Check sheet for the modelled part. Datum: model origin and axes. Units: mm. A direction names the side the tool comes from. Give positions to 0.01 mm unless a question says otherwise; leave off trailing zeros. Order: outer loops, then holes, each group sorted by start corner. A loop starts at its lowest first (then second) coordinate and runs counter-clockwise, first axis right, second up.
from build123d import *

# Parameters (mm, degrees)
F0_W      = 1600.2
F0_H      = 685.8
F1_DEPTH  = 19.05
F3_DEPTH  = 152.4
F5_DEPTH  = 152.4
F6_W      = 762
F6_H      = 19.05
F7_DEPTH  = 152.4
F8_W      = 381
F8_H      = 19.05
F9_DEPTH  = 152.4
F10_W     = 381
F10_H     = 19.05
F11_DEPTH = 152.4


with BuildPart() as f1:
    # F0 (on Front) → F1 (new body)
    with BuildSketch(Plane.XZ):
        with Locations((800.1, 342.9)):
            Rectangle(F0_W, F0_H)
    extrude(amount=F1_DEPTH)

    # F2 (on face) → F3 (join)
    with BuildSketch(Plane.XZ.offset(19.05)):
        Polygon((0, 685.8), (0, 0), (19.05, 0), (19.05, 666.75), (1581.15, 666.75), (1581.15, 0), (1600.2, 0), (1600.2, 685.8), align=None)
    extrude(amount=F3_DEPTH)

    # F4 (on face) → F5 (join)
    with BuildSketch(Plane.XZ.offset(19.05)):
        Polygon((419.1, 0), (419.1, 666.75), (400.05, 666.75), (400.05, 19.05), (19.05, 19.05), (19.05, 0), align=None)
        Polygon((1200.15, 666.75), (1181.1, 666.75), (1181.1, 0), (1581.15, 0), (1581.15, 19.05), (1200.15, 19.05), align=None)
    extrude(amount=F5_DEPTH)

    # F6 (on face) → F7 (join)
    with BuildSketch(Plane.XZ.offset(19.05)):
        with Locations((800.1, 466.725)):
            Rectangle(F6_W, F6_H)
    extrude(amount=F7_DEPTH)

    # F8 (on face) → F9 (join)
    with BuildSketch(Plane.XZ.offset(19.05)):
        with Locations((209.55, 454.025)):
            Rectangle(F8_W, F8_H)
        with Locations((209.55, 231.775)):
            Rectangle(F8_W, F8_H)
    extrude(amount=F9_DEPTH)

    # F10 (on face) → F11 (join)
    with BuildSketch(Plane.XZ.offset(19.05)):
        with Locations((1390.65, 454.025)):
            Rectangle(F10_W, F10_H)
        with Locations((1390.65, 231.775)):
            Rectangle(F10_W, F10_H)
    extrude(amount=F11_DEPTH)


solid = f1.part
1) Draft check along X on faces 1 (the face through (1388, -94, 666.75)), 2 (the face through (0, -85, 348)), 3 (the face through (789, 0, 348)). Enter one of: +X half, -X half, draft (parallel to the pull), parting line (faces both ways), or undercut.
Recorded:
face 1: undercut
face 2: -X half
face 3: draft
2) Section check B-B, the plane x = 367.5. Record the cut outline in (y, z), then the cut area to 3 significant figures.
Recorded:
outline: (-171.45, 0) - (0, 0) - (0, 685.8) - (-171.45, 685.8) - (-171.45, 666.75) - (-19.05, 666.75) - (-19.05, 463.55) - (-171.45, 463.55) - (-171.45, 444.5) - (-19.05, 444.5) - (-19.05, 241.3) - (-171.45, 241.3) - (-171.45, 222.25) - (-19.05, 222.25) - (-19.05, 19.05) - (-171.45, 19.05) - close
area: 24,700 mm2
3) Section check C-C, the plane y = -48.5. State how many separate pieces and enclosed holes the cut face has, then the cut area to 3 significant figures.
Recorded:
separate pieces: 1
enclosed holes: 7
area: 139,000 mm2
4) Set-up check for faces 4 (the face through (1581.15, -94, 122)), 5 (the face through (789, -8, 0)), 6 (the face through (1181.1, -94, 232)): record each of +Z, -Z, +X, -X, +Y, -Y from which the full face is reachable in a straight line by a thin tool's end or side.
Recorded:
face 4: -Y
face 5: -Z, +X, -X, +Y, -Y
face 6: -Z, -Y
5) Section check A-A, the plane z = 518. Record the cut outline in (x, y), then the cut area to 3 significant figures.
Recorded:
outline: (0, -171.45) - (19.05, -171.45) - (19.05, -19.05) - (400.05, -19.05) - (400.05, -171.45) - (419.1, -171.45) - (419.1, -19.05) - (1181.1, -19.05) - (1181.1, -171.45) - (1200.15, -171.45) - (1200.15, -19.05) - (1581.15, -19.05) - (1581.15, -171.45) - (1600.2, -171.45) - (1600.2, 0) - (0, 0) - close
area: 42,100 mm2
6) Depth check by flat-ended pin: pin 1 Ø5 at (y, z) = (-33, 355.5) entering from -X; pin 2 Ø4 at (x, z) = (996, 317) entering from -Y. Enter the tip coordinate at first touch or a pass-through.
Recorded:
pin 1: stops at x = 0
pin 2: stops at y = -19.05
7) Material ranges on L1, parallel to X at y = -32.5, z = 655.5; L2, parallel to Z at x = 1296, y = -129.5, recorded low to high.
Recorded:
L1: x = 0 to 19.05, 400.05 to 419.1, 1181.1 to 1200.15, 1581.15 to 1600.2
L2: z = 0 to 19.05, 222.25 to 241.3, 444.5 to 463.55, 666.75 to 685.8
8) Section check D-D, the plane x = 1018.5. Record the cut outline in (y, z), then the cut area to 3 significant figures.
Recorded:
outline: (-171.45, 457.2) - (-19.05, 457.2) - (-19.05, 0) - (0, 0) - (0, 685.8) - (-171.45, 685.8) - (-171.45, 666.75) - (-19.05, 666.75) - (-19.05, 476.25) - (-171.45, 476.25) - close
area: 18,900 mm2
